For this review, take the finished solid that the model builds, in its own axes (mm). A direction names the side the tool comes from. Round coordinates to 2 decimals unless told otherwise and drop trailing zeros. Loops run counter-clockwise (first coordinate to the right, second up) from the corner with the lowest first, then second, coordinate; pieces in that order, holes last. Notation, with made-up numbers: (21.25, -29) -> (71.25, -29) arc R19 cw to (71.25, -3) -> close; hole circle Ø8 at (9, 75). An arc over 180 degrees is marked (long way). Use one line per item in the form item = value. Start each with the question number.
Autodesk Inventor part; units mm, degrees
ref_plane "YZ Plane" through (0, 0, 0) normal (1, 0, 0) x (0, 1, 0)
ref_plane "XZ Plane" through (0, 0, 0) normal (0, 1, 0) x (-1, 0, 0)
sketch "Sketch2" plane through (0, 0, 0) normal (0, 0, 1) x (1, 0, 0)
  circle A0 centre (0, 0) radius 5
  dimension "d1" = 10
sketch "Sketch3" plane through (0, 0, 0) normal (0, 0, 1) x (1, 0, 0)
  circle A0 centre (0, 0) radius 3.1
  dimension "d2" = 6.2
sketch "Sketch4" plane through (0, 0, 0) normal (0, 0, 1) x (1, 0, 0)
  circle A0 centre (0, 0) radius 4.15
  dimension "d3" = 8.3
ref_plane "Work Plane5" through (0, 0, -10) normal (0, 0, 1) x (1, 0, 0)
sketch "Sketch5" plane through (0, 0, -10) normal (0, 0, 1) x (1, 0, 0)
  circle A0 centre (0, 0) radius 7.5055
  dimension "d9" = 15.011
ref_plane "Work Plane3" through (0, 0, -5) normal (0, 0, 1) x (1, 0, 0)
sketch "Sketch6" plane through (0, 0, -5) normal (0, 0, 1) x (1, 0, 0)
  circle A0 centre (0, 0) radius 6.75
  dimension "d11" = 13.5
loft "Loft1" add profiles "Sketch5", "Sketch6", "Sketch2"
extrude "Extrusion2" add sketch "Sketch4" along normal blind 0.5
extrude "Extrusion3" cut sketch "Sketch3" along normal blind 0.5 and the other way blind 10
ref_plane "Work Plane4" through (0, 0, -18) normal (0, 0, 1) x (1, 0, 0)
sketch "Sketch8" plane through (0, 0, -18) normal (0, 0, 1) x (1, 0, 0)
  line L0 (0, 7.5056) -> (6.5, 3.7528)
  line L1 (6.5, 3.7528) -> (6.5, -3.7528)
  line L2 (6.5, -3.7528) -> (0, -7.5056)
  line L3 (0, -7.5056) -> (-6.5, -3.7528)
  line L4 (-6.5, -3.7528) -> (-6.5, 3.7528)
  line L5 (-6.5, 3.7528) -> (0, 7.5056)
  point P0 (0, 0)
  point P1 (0, 0)
  dimension "d27" = 13
extrude "Extrusion4" add sketch "Sketch8" along normal blind 8
sketch "Sketch9" plane through (0, 0, -18) normal (0, 0, -1) x (-1, 0, 0)
  circle A0 centre (0, 0) radius 4
  dimension "d30" = 8
extrude "Extrusion5" add sketch "Sketch9" along normal blind 40
sketch "Sketch10" plane through (0, 0, -58) normal (0, 0, -1) x (-1, 0, 0)
  circle A0 centre (0, 0) radius 4
  circle A1 centre (0, 0) radius 1
  dimension "d33" = 2
extrude "Extrusion6" cut sketch "Sketch10" against normal blind 40 contours A1
sketch "Sketch11" plane through (0, 0, -18) normal (0, 0, -1) x (-1, 0, 0)
  circle A0 centre (0, 0) radius 4
  circle A1 centre (0, 0) radius 1
  dimension "d36" = 2
extrude "Extrusion7" cut sketch "Sketch11" against normal blind 8 contours A1
thread "Thread1"
fillet "Fillet1" radius 1.5 1 edges at (4, 0, -18)
properties part number "Adjustment screw"
Item 1: Draft analysis for pull direction Y (two halves, no side actions). For faces 5 (the cylindrical face through (-0.9, 4.05, 0.25)), 6 (the flat face through (3.2, 5.66, -14.06)), 7 (the cylindrical face through (1.43, 2.75, -4.82)), 8 (the flat face through (6.5, 0, -14)), state which applies: +Y half, -Y half, draft (parallel to the pull), parting line (faces both ways), or undercut.
Item 2: For P1, Ø0.8, axis at x = 7, y = 0.5, coming from the -Z side; P2, Ø1.9, axis at x = -1, y = 0.5, coming from the +Z side; P3, Ø6, axis at y = -2, z = -16, coming from the -X side, all flat-tipped, find the tip position at first contact; note any pin that passes through.
Item 3: Machinability: for faces 1 (the flat face through (7, 0, -10)), 2 (the cylindrical face through (0.867, 3.905, -38.48)), 3 (the flat face through (-3.2, -5.66, -14.06)), 4 (the flat face through (3.3, -5.6, -14.1)), which of the approach directions +Z, -Z, +X, -X, +Y, -Y give a long, thin tool a straight path to every point of the face, cutting with its end or side? Answer none if there is none.
Item 4: Take a section at A-A on z = -16.5. Give the boundary of the cut face in (x, y), plus the area to 3 significant figures.
Item 5: Wall thickness on line 1 (Y direction, x = 0, z = -38.5); line 2 (Y direction, x = 0, z = -3.5); line 3 (X direction, y = -0.5, z = -5.5): over which ranges is each line inside the solid? List them lowest first.
Item 6: Take a section at B-B on z = -52. Give the boundary of the cut face in (x, y), plus the area to 3 significant figures.
Results:
q1.face_5 = parting line
q1.face_6 = +Y half
q1.face_7 = undercut
q1.face_8 = draft
q2.P1 = -10
q2.P2 = -10
q2.P3 = -6.5
q3.face_1 = -Z, +X, +Y, -Y
q3.face_2 = -Z
q3.face_3 = -Z, -X, -Y
q3.face_4 = -Z, +X, -Y
q4.outline = (-6.5, -3.75) -> (0, -7.51) -> (6.5, -3.75) -> (6.5, 3.75) -> (0, 7.51) -> (-6.5, 3.75) -> close; hole circle Ø2 at (0, 0)
q4.area = 143 mm2
q5.line_1 = -4 to -1, 1 to 4
q5.line_2 = -6.34 to -3.1, 3.1 to 6.34
q5.line_3 = -6.85 to -3.06, 3.06 to 6.85
q6.outline = circle Ø8 at (0, 0); hole circle Ø2 at (0, 0)
q6.area = 47.1 mm2
